Autodesk Inventor part; units mm, degrees
ref_plane "YZ Plane" through (0, 0, 0) normal (1, 0, 0) x (0, 1, 0)
ref_plane "XZ Plane" through (0, 0, 0) normal (0, 1, 0) x (-1, 0, 0)
ref_plane "XY Plane" through (0, 0, 0) normal (0, 0, 1) x (1, 0, 0)
sketch "Sketch1" plane through (0, 0, 0) normal (1, 0, 0) x (0, 1, 0)
  line L0 (0, 0) -> (488.95, 0)
  line L1 (488.95, -406.4) -> (0, -406.4)
  line L2 (0, -406.4) -> (0, 0)
  line L3 (488.95, 0) -> (488.95, -165.1)
  line L4 (488.95, -165.1) -> (412.75, -165.1)
  line L5 (412.75, -165.1) -> (412.75, -215.9)
  line L6 (412.75, -215.9) -> (488.95, -215.9)
  line L7 (488.95, 0) -> (488.95, -165.1)
  line L8 (488.95, -215.9) -> (488.95, -406.4)
  line L9 (346.075, 3.175) -> (342.9, 3.175)
  line L10 (342.9, 3.175) -> (346.075, 3.175)
  line L11 (358.775, 3.175) -> (361.95, 3.175)
  line L12 (374.65, 3.175) -> (377.825, 3.175)
  line L13 (390.525, 3.175) -> (393.7, 3.175)
  line L14 (98.425, -406.4) -> (3.175, -406.4)
  line L15 (457.2, 0) -> (0, 0)
  line L16 (3.175, 0) -> (98.425, 0)
  line L17 (0, -406.4) -> (3.175, -406.4)
  dimension "d9" = 3.175
extrude "Extrusion1" add sketch "Sketch1" along normal blind 3.175
sketch "Sketch2" plane through (0, 0, 0) normal (-1, 0, 0) x (0, 0, 1)
  line L0 (-406.4, 0) -> (-406.4, 488.95)
  line L1 (0, 0) -> (-406.4, 0)
  line L2 (0, 488.95) -> (0, 0)
  line L3 (-165.1, 488.95) -> (0, 488.95)
  line L4 (-165.1, 412.75) -> (-165.1, 488.95)
  line L5 (-215.9, 412.75) -> (-165.1, 412.75)
  line L6 (-215.9, 488.95) -> (-215.9, 412.75)
  line L7 (-406.4, 488.95) -> (-215.9, 488.95)
  line L8 (-339.725, 53.1114) -> (-339.725, 13.1826)
  line L9 (-279.781, 13.1826) -> (-279.781, 53.1114)
  line L10 (-289.7886, 63.119) -> (-329.7174, 63.119)
  circle A0 centre (-334.7212, 58.1152) radius 2.159
  circle A1 centre (-284.7848, 58.1152) radius 2.159
  circle A2 centre (-334.7212, 8.1788) radius 2.159
  circle A3 centre (-284.7848, 8.1788) radius 2.159
  line L11 (-329.7174, 63.119) -> (-329.7174, 53.1114)
  line L12 (-329.7174, 53.1114) -> (-339.725, 53.1114)
  line L13 (-289.7886, 63.119) -> (-289.7886, 53.1114)
  line L14 (-289.7886, 53.1114) -> (-279.781, 53.1114)
  line L15 (-329.7174, 3.175) -> (-329.7174, 13.1826)
  line L16 (-329.7174, 13.1826) -> (-339.725, 13.1826)
  line L17 (-289.7886, 3.175) -> (-289.7886, 13.1826)
  line L18 (-289.7886, 13.1826) -> (-279.781, 13.1826)
  line L19 (-212.725, 63.1698) -> (-178.2826, 63.1698)
  circle A4 centre (-219.3036, 56.7436) radius 2.54
  circle A5 centre (-219.3036, 9.6012) radius 2.54
  circle A6 centre (-172.1612, 56.7436) radius 2.54
  circle A7 centre (-172.1612, 9.6012) radius 2.54
  line L20 (-136.9822, 10.6172) -> (-158.4706, 10.6172)
  line L21 (-158.4706, 15.6972) -> (-136.9822, 15.6972)
  arc A8 (-136.9822, 10.6172) -> (-136.9822, 15.6972) centre (-136.9822, 13.1572) ccw
  arc A9 (-158.4706, 15.6972) -> (-158.4706, 10.6172) centre (-158.4706, 13.1572) ccw
  line L22 (-136.9822, 20.5994) -> (-158.4706, 20.5994)
  line L23 (-158.4706, 25.6794) -> (-136.9822, 25.6794)
  arc A10 (-136.9822, 20.5994) -> (-136.9822, 25.6794) centre (-136.9822, 23.1394) ccw
  arc A11 (-158.4706, 25.6794) -> (-158.4706, 20.5994) centre (-158.4706, 23.1394) ccw
  line L24 (-136.9822, 30.5816) -> (-158.4706, 30.5816)
  line L25 (-158.4706, 35.6616) -> (-136.9822, 35.6616)
  arc A12 (-136.9822, 30.5816) -> (-136.9822, 35.6616) centre (-136.9822, 33.1216) ccw
  arc A13 (-158.4706, 35.6616) -> (-158.4706, 30.5816) centre (-158.4706, 33.1216) ccw
  line L26 (-136.9822, 40.5638) -> (-158.4706, 40.5638)
  line L27 (-158.4706, 45.6438) -> (-136.9822, 45.6438)
  arc A14 (-136.9822, 40.5638) -> (-136.9822, 45.6438) centre (-136.9822, 43.1038) ccw
  arc A15 (-158.4706, 45.6438) -> (-158.4706, 40.5638) centre (-158.4706, 43.1038) ccw
  line L28 (-136.9822, 50.546) -> (-158.4706, 50.546)
  line L29 (-158.4706, 55.626) -> (-136.9822, 55.626)
  arc A16 (-136.9822, 50.546) -> (-136.9822, 55.626) centre (-136.9822, 53.086) ccw
  arc A17 (-158.4706, 55.626) -> (-158.4706, 50.546) centre (-158.4706, 53.086) ccw
  line L30 (-212.725, 63.1698) -> (-212.725, 50.4698)
  line L31 (-212.725, 50.4698) -> (-219.3036, 50.4698)
  line L32 (-172.1612, 50.4698) -> (-178.2826, 50.4698)
  line L33 (-178.2826, 50.4698) -> (-178.2826, 63.1698)
  line L34 (-178.2826, 3.3274) -> (-178.2826, 16.0274)
  line L35 (-178.2826, 16.0274) -> (-172.1612, 16.0274)
  line L36 (-219.3036, 16.0274) -> (-212.725, 16.0274)
  line L37 (-212.725, 16.0274) -> (-212.725, 3.3274)
  line L38 (-219.3036, 50.4698) -> (-219.3036, 16.0274)
  line L39 (-172.1612, 50.4698) -> (-172.1612, 16.0274)
  line L40 (-403.225, 3.175) -> (-339.725, 3.175)
  line L41 (-329.7174, 3.175) -> (-289.7886, 3.175)
  line L42 (53.975, 3.175) -> (-403.225, 3.175)
  line L43 (-178.2826, 6.0198) -> (-178.2826, 0)
  line L44 (-178.2826, 0) -> (-212.725, 0)
  line L45 (-212.725, 0) -> (-212.725, 6.0198)
  line L46 (-406.4, 0) -> (-406.4, 488.95)
  line L47 (-406.4, 0) -> (-406.4, 3.175)
  line L48 (-406.4, 0) -> (-403.225, 0)
  line L49 (-403.225, 0) -> (-403.225, 3.175)
  line L50 (-403.225, 3.175) -> (-406.4, 3.175)
  line L51 (-406.4, 3.175) -> (-406.4, 0)
  point P0 (-332.8924, 0)
  point P1 (-292.9636, 0)
  point P2 (-212.725, 0)
  point P3 (-178.2826, 0)
  point P4 (-212.725, 3.175)
  point P5 (-178.2826, 3.175)
  dimension "d12" = 3.175
  dimension "d15" = 3.175
  dimension "d16" = 3.175
extrude "Extrusion3" cut sketch "Sketch2" against normal blind 25.4 contours L45 L37 L36 L38 L31 L30 L19 L33 L32 L39 L35 L34 L43 L42 | L15 L16 L8 L12 L11 L10 L13 L14 L9 L18 L17 L41 | A0 | A1 | A2 | A3 | A4 | A5 | A6 | A7 | L20 A9 L21 A8 | L22 A11 L23 A10 | L24 A13 L25 A12 | L26 A15 L27 A14 | L28 A17 L29 A16
properties part number "220310 Left Side"
CAD build for the part. Positions are in the model's coordinates, mm. Coordinates: 2 decimals unless noted, no trailing zeros. Write each loop counter-clockwise with the first axis right and the second up, starting at its lowest first coordinate (ties: lowest second). Pieces come first, ordered by that corner, then holes. Notation, with made-up numbers: M 33.25,-36 L 55.25,-36 A29 ccw 55.25,-10 Z; hole C 67.5,18 d6. An arc over 180 degrees is marked long. Return JSON: item names as keys, results as strings.
Item 1: Slice it at B-B, the plane x = 2.5. State how many separate pieces and enclosed holes the cut face has, and give its area (3 significant figures).
Findings below:
{"separate pieces": "1", "enclosed holes": "15", "area": "188,000 mm2"}
Item 2: Drop flat-ended pins along their axis: pin 1 Ø5.5 at (y, z) = (8.18, -284.78) entering from -X; pin 2 Ø1.5 at (x, z) = (2, -214.5) entering from +Y. Give the stop position or say it passes through.
Findings below:
{"pin 1": "stops at x = 0", "pin 2": "stops at y = 412.75"}
Item 3: Probe line 1 (Y direction, x = 0.5, z = -318) (3 decimals); line 2 (Z direction, x = 0.9, y = 466); line 3 (Y direction, x = 0.75, z = -333). List the from-to ranges inside material, lowest first. Write a range as from..to.
Findings below:
{"line 1": "y = 0..3.175, 63.119..488.95", "line 2": "z = -406.4..-215.9, -165.1..0", "line 3": "y = 0..6.88, 9.48..13.18, 53.11..56.81, 59.42..488.95"}
Item 4: Slice it at A-A, the plane z = -151.5. Write the cut outline in (x, y) (3 decimals).
Findings below:
{"outline": "M 0,0 L 3.175,0 L 3.175,10.617 L 0,10.617 Z; M 0,15.697 L 3.175,15.697 L 3.175,20.599 L 0,20.599 Z; M 0,25.679 L 3.175,25.679 L 3.175,30.582 L 0,30.582 Z; M 0,35.662 L 3.175,35.662 L 3.175,40.564 L 0,40.564 Z; M 0,45.644 L 3.175,45.644 L 3.175,50.546 L 0,50.546 Z; M 0,55.626 L 3.175,55.626 L 3.175,488.95 L 0,488.95 Z"}
